from build123d import *

# Parameters (mm, degrees)
PAD_DEPTH         = 3.9
SKETCH001_R       = 6
PAD001_DEPTH      = 7.8
FILLET_R          = 3.5
SKETCH002_R       = 1.75
POCKET_DEPTH      = 4.001
POCKET_DEPTH_BACK = 21.001
POCKET001_DEPTH   = 4
SKETCH004_R       = 3
POCKET002_DEPTH   = 6


with BuildPart() as part:
    # Sketch → Pad (new body, symmetric)
    with BuildSketch(Plane.XY):
        with BuildLine():
            Line((-3.9, 0), (3.9, 0))
            Line((3.9, 0), (3.9, 0.8))
            Line((3.9, 0.8), (5.35, 0.8))
            ThreePointArc((5.35, 0.8), (0, 4), (-5.35, 0.8))
            Line((-5.35, 0.8), (-3.9, 0.8))
            Line((-3.9, 0.8), (-3.9, 0))
        make_face()
    extrude(amount=PAD_DEPTH, both=True)

    # Sketch001 (on Face7 of Pad) → Pad001 (join)
    with BuildSketch(Plane(origin=(0, 0, -3.9), x_dir=(1, 0, 0), z_dir=(0, 0, -1))):
        with BuildLine():
            ThreePointArc((3.9, 3.888896), (0, 21), (-3.9, 3.888896))
            Line((-3.9, 3.888896), (-3.9, 0))
            Line((-3.9, 0), (3.9, 0))
            Line((3.9, 0), (3.9, 3.888896))
        make_face()
        with Locations((0, 12)):
            Circle(SKETCH001_R, mode=Mode.SUBTRACT)
    extrude(amount=-PAD001_DEPTH)

    # Fillet
    fillet_edges = [part.edges().sort_by_distance(p)[0] for p in [
        (-3.9, -1.944448, -3.9),
        (-3.9, -1.944448, 3.9),
        (3.9, -1.944448, 3.9),
        (3.9, -1.944448, -3.9),
    ]]
    fillet(fillet_edges, radius=FILLET_R)

    # Sketch002 → Pocket (cut, two sides)
    with BuildSketch(Plane.XZ) as pocket_sk:
        Circle(SKETCH002_R)
    extrude(amount=-POCKET_DEPTH, mode=Mode.SUBTRACT)
    extrude(pocket_sk.sketch, amount=POCKET_DEPTH_BACK, mode=Mode.SUBTRACT)

    # Sketch003 (on DatumPlane) → Pocket001 (cut)
    with BuildSketch(Plane.XZ.offset(-4)):
        Polygon((-1.45, -2.511474), (1.45, -2.511474), (2.9, 0), (1.45, 2.511474), (-1.45, 2.511474), (-2.9, 0), align=None)
    extrude(amount=POCKET001_DEPTH, mode=Mode.SUBTRACT)

    # Sketch004 (on DatumPlane) → Pocket002 (cut)
    with BuildSketch(Plane.XZ.offset(3)):
        Circle(SKETCH004_R)
    extrude(amount=POCKET002_DEPTH, mode=Mode.SUBTRACT)


solid = part.part
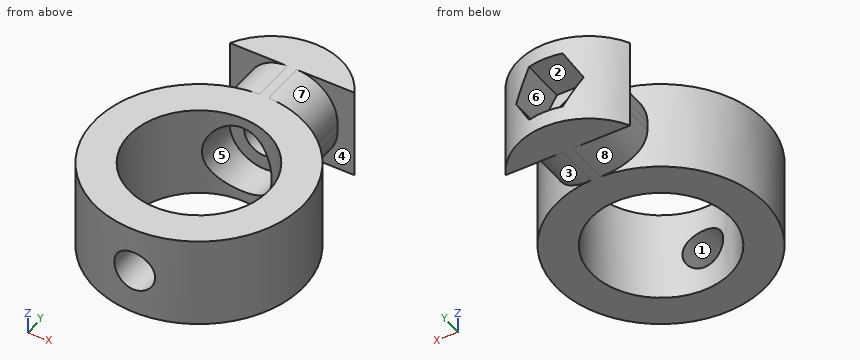
The listing builds one solid part. Answer for the finished solid, in the listing's coordinates (mm). Face numbers are marked on the shaded views. A direction names the side the tool comes from. Coordinates: 2 decimals unless noted, no trailing zeros. Loops run counter-clockwise (first coordinate to the right, second up) from the corner with the lowest first, then second, coordinate; pieces in that order, holes last. Notation, with made-up numbers: M 54.25,-28 L 69.25,-28 A30 cw 69.25,-4 Z; hole C -4,-21 d10. An arc over 180 degrees is marked long. Answer in a Markdown table with one row per item.
1) Find section D-D (z = 2.25). Determine the outline of the cut face in (x, y).
Answers below:
| item | result |
|---|---|
| outline | M -5.35,0.8 L -3.37,0.8 L -3.37,-3.66 A9 ccw long 3.37,-3.66 L 3.37,0.8 L 5.35,0.8 A6.07 ccw 1.6,3.79 L 1.6,0 L -1.6,0 L -1.6,3.79 A6.07 ccw Z; hole M -1.98,-6.34 A6 ccw long 1.98,-6.34 L 1.98,-3 L -1.98,-3 Z |
2) Determine the mould class of the marked faces 1, 2, 3 and 4 for opening direction Z: released by +Z, released by -Z, zero draft, split by the parting line, or undercut.
Answers below:
| item | result |
|---|---|
| face 1 | undercut |
| face 2 | undercut |
| face 3 | released by -Z |
| face 4 | zero draft |
3) Find section A-A (y = -12). Determine the outline of the cut face in (x, z), then the cut area to 3 significant figures.
Answers below:
| item | result |
|---|---|
| outline | M -9,-3.9 L -6,-3.9 L -6,3.9 L -9,3.9 Z; M 6,-3.9 L 9,-3.9 L 9,3.9 L 6,3.9 Z |
| area | 46.8 mm^2 |
4) Which of the six approach directions +Z, -Z, +X, -X, +Y, -Y give full straight-line access (tool end or side, diameter ignored) to the marked faces 5, 6, 7 and 8?
Answers below:
| item | result |
|---|---|
| face 5 | none |
| face 6 | +Y |
| face 7 | +Z, +X |
| face 8 | -Z, -X |
5) Find the intervals of material crossed by probe 1 along Z at (x, y) = (0, -19.05); probe 2 along X at (y, z) = (-12, 1.25); probe 3 along X at (y, z) = (-3.8, 0), in increasing order.
Answers below:
| item | result |
|---|---|
| probe 1 | -3.9 to -1.75, 1.75 to 3.9 |
| probe 2 | -9 to -6, 6 to 9 |
| probe 3 | -3.9 to -3, 3 to 3.9 |
6) Find section C-C (x = 4.25). Determine the outline of the cut face in (y, z), then the cut area to 3 significant figures.
Answers below:
| item | result |
|---|---|
| outline | M -19.93,-3.9 L -16.24,-3.9 L -16.24,3.9 L -19.93,3.9 Z; M -7.76,-3.9 L -4.07,-3.9 L -4.07,3.9 L -7.76,3.9 Z; M 0.8,-3.9 L 2.26,-3.9 L 2.26,3.9 L 0.8,3.9 Z |
| area | 69.1 mm^2 |
7) Find section B-B (x = 0). Determine the outline of the cut face in (y, z), then the cut area to 3 significant figures.
Answers below:
| item | result |
|---|---|
| outline | M -21,-3.9 L -18,-3.9 L -18,-1.75 L -21,-1.75 Z; M -21,1.75 L -18,1.75 L -18,3.9 L -21,3.9 Z; M -6,-3.9 L 4,-3.9 L 4,-2.51 L 0,-2.51 L 0,-1.75 L -3,-1.75 L -3,-3 L -6,-3 Z; M -6,3 L -3,3 L -3,1.75 L 0,1.75 L 0,2.51 L 4,2.51 L 4,3.9 L -6,3.9 Z |
| area | 42.3 mm^2 |
8) Given pin 1 (0.9 mm diameter, centred on y = -0.5, z = 0, fed in from -X); pin 2 (2 mm diameter, centred on y = -10, z = -1, fed in from -X); pin 3 (2 mm diameter, centred on y = -6, z = 2.5, fed in from +X), each flat-ended and moving along its own axis, determine where each tip first touches the part or whether it passes through.
Answers below:
| item | result |
|---|---|
| pin 1 | x = -3.9 |
| pin 2 | x = -8.94 |
| pin 3 | x = 7.48 |
